Here's how the part is built. I have some questions about the finished solid (model axes, mm). A direction names the side the tool comes from. Round coordinates to 2 decimals unless told otherwise and drop trailing zeros. Write each loop counter-clockwise with the first axis right and the second up, starting at its lowest first coordinate (ties: lowest second). Pieces come first, ordered by that corner, then holes. Notation, with made-up numbers: (-9, -23.5) - (19, -23.5) arc R25 cw to (19, 14.5) - close; hole circle Ø11 at (-5, 9). An arc over 180 degrees is marked (long way). One line per item, written item: value. Start each with the question number.
Item 1: For P1, Ø4, axis at y = 30.5, z = 20, coming from the +X side; P2, Ø3, axis at x = 45, z = -15.5, coming from the -Y side; P3, Ø8, axis at y = 21.5, z = 27.5, coming from the -X side; P4, Ø3, axis at x = -3.5, z = 24, coming from the +Y side, each with a flat end and sliding along its axis, tell me the tip position at first contact or that it passes through.
Item 2: Imagine slicing it at B-B, the plane y = 35. Please give me the cut outline in (x, z).
Item 3: Thinking about a two-plate mould opening in X: for faces 3 (the face through (67, 22, 0)), 4 (the face through (-1, 23, -33.5)), 5 (the face through (-67, 22, 0)), 6 (the face through (-1, 2, 0)), which applies, released by +X, released by -X, zero draft, split by the parting line, or undercut?
Item 4: For faces 1 (the face through (-1, 22, -35)), 2 (the face through (65.5, 23, 0)), which set-ups out of +Z, -Z, +X, -X, +Y, -Y let a thin tool reach every point of the face, with its end or its side?
Item 5: If I drill on line 1 (Z direction, x = -15.5, y = 37.5); line 2 (X direction, y = 3, z = 14); line 3 (Y direction, x = -19, z = -16.5), over which ranges is the centre line in solid material (lowest first)?
```python
from build123d import *

# Parameters (mm, degrees)
SKETCH_1_W          = 134
SKETCH_1_H          = 70
EXTRUDE_1_DEPTH     = 45
SKETCH_2_W          = 131
SKETCH_2_H          = 67
CUT_EXTRUDE_1_DEPTH = 43
FILLET_1_R          = 20
FILLET_2_R          = 0.75


with BuildPart() as part:
    # 草图1 → 凸台-拉伸1 (new body)
    with BuildSketch(Plane(origin=(0, 0, 0), x_dir=(1, 0, 0), z_dir=(0, 1, 0))):
        Rectangle(SKETCH_1_W, SKETCH_1_H)
    extrude(amount=EXTRUDE_1_DEPTH)

    # 草图2 → 切除-拉伸1 (cut)
    with BuildSketch(Plane(origin=(0, 45, 0), x_dir=(1, 0, 0), z_dir=(0, 1, 0))):
        Rectangle(SKETCH_2_W, SKETCH_2_H)
    extrude(amount=-CUT_EXTRUDE_1_DEPTH, mode=Mode.SUBTRACT)

    # 圆角1
    fillet_1_edges = [part.edges().sort_by_distance(p)[0] for p in [
        (-65.5, 23.5, 33.5),
        (65.5, 23.5, 33.5),
        (65.5, 23.5, -33.5),
        (-65.5, 23.5, -33.5),
        (-67, 22.5, 35),
        (67, 22.5, 35),
        (67, 22.5, -35),
        (-67, 22.5, -35),
    ]]
    fillet(fillet_1_edges, radius=FILLET_1_R)

    # 圆角2
    fillet_2_edges = [part.edges().sort_by_distance(p)[0] for p in [
        (0, 45, 33.5),
        (-65.5, 45, 0),
        (0, 45, 35),
        (-67, 45, 0),
        (0, 45, -35),
        (0, 45, -33.5),
        (65.5, 45, 0),
        (67, 45, 0),
        (-59.642135624, 45, 27.642135624),
        (-59.642135624, 45, -27.642135624),
        (59.642135624, 45, -27.642135624),
        (59.642135624, 45, 27.642135624),
        (61.142135624, 45, -29.142135624),
        (61.142135624, 45, 29.142135624),
        (-61.142135624, 45, -29.142135624),
        (-61.142135624, 45, 29.142135624),
    ]]
    fillet(fillet_2_edges, radius=FILLET_2_R - 0.0001)  # a hair under: the kernel refuses the full size


solid = part.part
```
Values follow:
1. P1: stops at x = 66.77
1. P2: stops at y = 0
1. P3: stops at x = -65.1
1. P4: stops at y = 2
2. outline: (-67, -15) arc R20 ccw to (-47, -35) - (47, -35) arc R20 ccw to (67, -15) - (67, 15) arc R20 ccw to (47, 35) - (-47, 35) arc R20 ccw to (-67, 15) - close; hole (-65.5, -13.5) arc R20 ccw to (-45.5, -33.5) - (45.5, -33.5) arc R20 ccw to (65.5, -13.5) - (65.5, 13.5) arc R20 ccw to (45.5, 33.5) - (-45.5, 33.5) arc R20 ccw to (-65.5, 13.5) - close
3. face 3: released by +X
3. face 4: undercut
3. face 5: released by -X
3. face 6: undercut
4. face 1: -Z, +X, -X, +Y, -Y
4. face 2: +Y
5. line 1: z = -35 to -33.5, 33.5 to 35
5. line 2: x = -67 to -65.49, 65.49 to 67
5. line 3: y = 0 to 2
